```python
from build123d import *

# Parameters (mm, degrees)
SKETCH_1_R          = 10.25
SKETCH_1_R_2        = 1.6
EXTRUDE_1_DEPTH     = 10
SKETCH_3_R          = 1.65
CUT_EXTRUDE_2_DEPTH = 10
FILLET_1_R          = 2
CUT_EXTRUDE_START   = -5
SKETCH_4_R          = 1.6
CUT_EXTRUDE_3_DEPTH = 5
FILLET_2_R          = 2


with BuildPart() as part:
    # ｽｹｯﾁ1 → ﾎﾞｽ - 押し出し1 (new body)
    with BuildSketch(Plane.XY):
        with BuildLine():
            Line((-25, -15), (-19.25171886, 5.419531433))
            ThreePointArc((-19.25171886, 5.419531433), (-15.334292097, 12.83976191), (-8.717797887, 18))
            Line((-8.717797887, 18), (8.717797887, 18))
            ThreePointArc((8.717797887, 18), (15.334292097, 12.83976191), (19.25171886, 5.419531433))
            Line((19.25171886, 5.419531433), (25, -15))
            Line((25, -15), (25, -25))
            Line((25, -25), (-25, -25))
            Line((-25, -25), (-25, -15))
        make_face()
        Circle(SKETCH_1_R, mode=Mode.SUBTRACT)
        with Locations((9.192388155, 9.192388155)):
            Circle(SKETCH_1_R_2, mode=Mode.SUBTRACT)
        with Locations((9.192388155, -9.192388155)):
            Circle(SKETCH_1_R_2, mode=Mode.SUBTRACT)
        with Locations((-9.192388155, -9.192388155)):
            Circle(SKETCH_1_R_2, mode=Mode.SUBTRACT)
        with Locations((-9.192388155, 9.192388155)):
            Circle(SKETCH_1_R_2, mode=Mode.SUBTRACT)
    extrude(amount=EXTRUDE_1_DEPTH)

    # ｽｹｯﾁ3 → ｶｯﾄ - 押し出し2 (cut)
    with BuildSketch(Plane.XZ.offset(25)):
        with Locations(Location((-20, 5, 0), (0, 0, 270))):
            Circle(SKETCH_3_R)
        with Locations(Location((20, 5, 0), (0, 0, 90))):
            Circle(SKETCH_3_R)
    extrude(amount=-CUT_EXTRUDE_2_DEPTH, mode=Mode.SUBTRACT)

    # ﾌｨﾚｯﾄ1
    fillet_1_edges = [part.edges().sort_by_distance(p)[0] for p in [
        (25, -25, 5),
        (-25, -25, 5),
        (-25, -15, 5),
        (-8.717797887, 18, 5),
        (8.717797887, 18, 5),
        (25, -15, 5),
    ]]
    fillet(fillet_1_edges, radius=FILLET_1_R)

    # ｽｹｯﾁ4 → ｶｯﾄ - 押し出し3 (cut)
    with BuildSketch(Plane.XY.offset(10).offset(CUT_EXTRUDE_START)):
        with BuildLine():
            ThreePointArc((12.365702043, 8.49054845), (11.490485194, 11.490485194), (8.49054845, 12.365702043))
            ThreePointArc((8.49054845, 12.365702043), (0, 15), (-8.49054845, 12.365702043))
            ThreePointArc((-8.49054845, 12.365702043), (-11.490485194, 11.490485194), (-12.365702043, 8.49054845))
            ThreePointArc((-12.365702043, 8.49054845), (-15, 0), (-12.365702043, -8.49054845))
            ThreePointArc((-12.365702043, -8.49054845), (-11.490485194, -11.490485194), (-8.49054845, -12.365702043))
            ThreePointArc((-8.49054845, -12.365702043), (0, -15), (8.49054845, -12.365702043))
            ThreePointArc((8.49054845, -12.365702043), (11.490485194, -11.490485194), (12.365702043, -8.49054845))
            ThreePointArc((12.365702043, -8.49054845), (15, 0), (12.365702043, 8.49054845))
        make_face()
        with Locations((9.192388155, 9.192388155)):
            Circle(SKETCH_4_R, mode=Mode.SUBTRACT)
    extrude(amount=CUT_EXTRUDE_3_DEPTH, mode=Mode.SUBTRACT)

    # ﾌｨﾚｯﾄ2
    fillet_2_edges = [part.edges().sort_by_distance(p)[0] for p in [
        (-8.49054845, 12.365702043, 7.5),
        (8.49054845, 12.365702043, 7.5),
        (12.365702043, 8.49054845, 7.5),
        (12.365702043, -8.49054845, 7.5),
        (8.49054845, -12.365702043, 7.5),
        (-8.49054845, -12.365702043, 7.5),
        (-12.365702043, -8.49054845, 7.5),
        (-12.365702043, 8.49054845, 7.5),
    ]]
    fillet(fillet_2_edges, radius=FILLET_2_R)


solid = part.part
```
Source: CAD feature listing. Evaluate the final solid. Frame: model axes, mm. A direction names the side the tool comes from. Give positions to 0.01 mm unless a question says otherwise; leave off trailing zeros. Loops run counter-clockwise (first coordinate to the right, second up) from the corner with the lowest first, then second, coordinate; pieces in that order, holes last. Notation, with made-up numbers: (18, -6.5) -> (74, -6.5) arc R12 ccw to (74, 2.5) -> close; hole circle Ø11 at (85, 3). An arc over 180 degrees is marked (long way). Put each result on its own line as item: value. Start each with the question number.
1) Draft query along Z for faces 4 (the face through (-18.364, -20.07, 5.215)), 5 (the face through (0, 18, 5)), 6 (the face through (10, -3, 5)). Return one class per face: released by +Z, released by -Z, zero draft, split by the parting line, or undercut.
2) Material intervals for probe 1 along X at (y, z) = (9, 3); probe 2 along X at (y, z) = (-23, 6.25); probe 3 along Z at (x, y) = (20, -21.5), sorted ascending.
3) Cut plane A-A (x = 0). Return loops of the section in (y, z), then the cut area to 4 significant figures.
4) Contact query for flat-ended pins moving along their axis: P1, Ø3, axis at y = -11, z = 2.5, coming from the -X side; P2, Ø1.9, axis at x = -9.19, y = 9.19, coming from the +Z side; P3, Ø5, axis at x = 9.19, y = 9.19, coming from the +Z side; P4, Ø5.5, axis at x = -20, z = 5, coming from the +Y side. Output: stop coordinate, or through.
5) Cut plane B-B (y = 0). Return loops of the section in (x, z).
6) Cut plane C-C (y = -17.5). Return loops of the section in (x, z), then the cut area to 3 significant figures.
7) Cut plane D-D (z = 4.25). Return loops of the section in (x, y).
8) Reachability of faces 1 (the face through (15.42, 12.737, 4.93)), 2 (the face through (20, -15, 5)), 3 (the face through (0, 15, 7)) from +Z, -Z, +X, -X, +Y, -Y: full face, straight path, thin tool, end or side. Return the list, or none.
Results are:
1. face 4: undercut
1. face 5: zero draft
1. face 6: released by +Z
2. probe 1: x = -17.86 to -10.78, -7.6 to -4.91, 4.91 to 7.6, 10.78 to 17.86
2. probe 2: x = -25 to -21.08, -18.92 to 18.92, 21.08 to 25
2. probe 3: z = 0 to 3.35, 6.65 to 10
3. outline: (-25, 0) -> (-10.25, 0) -> (-10.25, 5) -> (-15, 5) -> (-15, 10) -> (-25, 10) -> close; (10.25, 0) -> (18, 0) -> (18, 10) -> (15, 10) -> (15, 5) -> (10.25, 5) -> close
3. area: 177.5 mm2
4. P1: stops at x = -24.3
4. P2: passes through
4. P3: stops at z = 5
4. P4: stops at y = 10.12
5. outline: (-20.78, 0) -> (-10.25, 0) -> (-10.25, 5) -> (-15, 5) -> (-15, 10) -> (-20.78, 10) -> close; (10.25, 0) -> (20.78, 0) -> (20.78, 10) -> (15, 10) -> (15, 5) -> (10.25, 5) -> close
6. outline: (-25, 0) -> (25, 0) -> (25, 10) -> (-25, 10) -> close; hole circle Ø3.3 at (-20, 5); hole circle Ø3.3 at (20, 5)
6. area: 483 mm2
7. outline: (-25, -23) arc R2 ccw to (-23, -25) -> (-21.47, -25) -> (-21.47, -15) -> (-18.53, -15) -> (-18.53, -25) -> (18.53, -25) -> (18.53, -15) -> (21.47, -15) -> (21.47, -25) -> (23, -25) arc R2 ccw to (25, -23) -> (25, -15.28) arc R2 ccw to (24.93, -14.73) -> (19.25, 5.42) arc R20 ccw to (9.16, 17.78) arc R2 ccw to (8.25, 18) -> (-8.25, 18) arc R2 ccw to (-9.16, 17.78) arc R20 ccw to (-19.25, 5.42) -> (-24.93, -14.73) arc R2 ccw to (-25, -15.28) -> close; hole circle Ø3.2 at (-9.19, -9.19); hole circle Ø3.2 at (-9.19, 9.19); hole circle Ø20.5 at (0, 0); hole circle Ø3.2 at (9.19, -9.19); hole circle Ø3.2 at (9.19, 9.19)
8. face 1: +Z, -Z, +X, +Y
8. face 2: -Y
8. face 3: +Z
